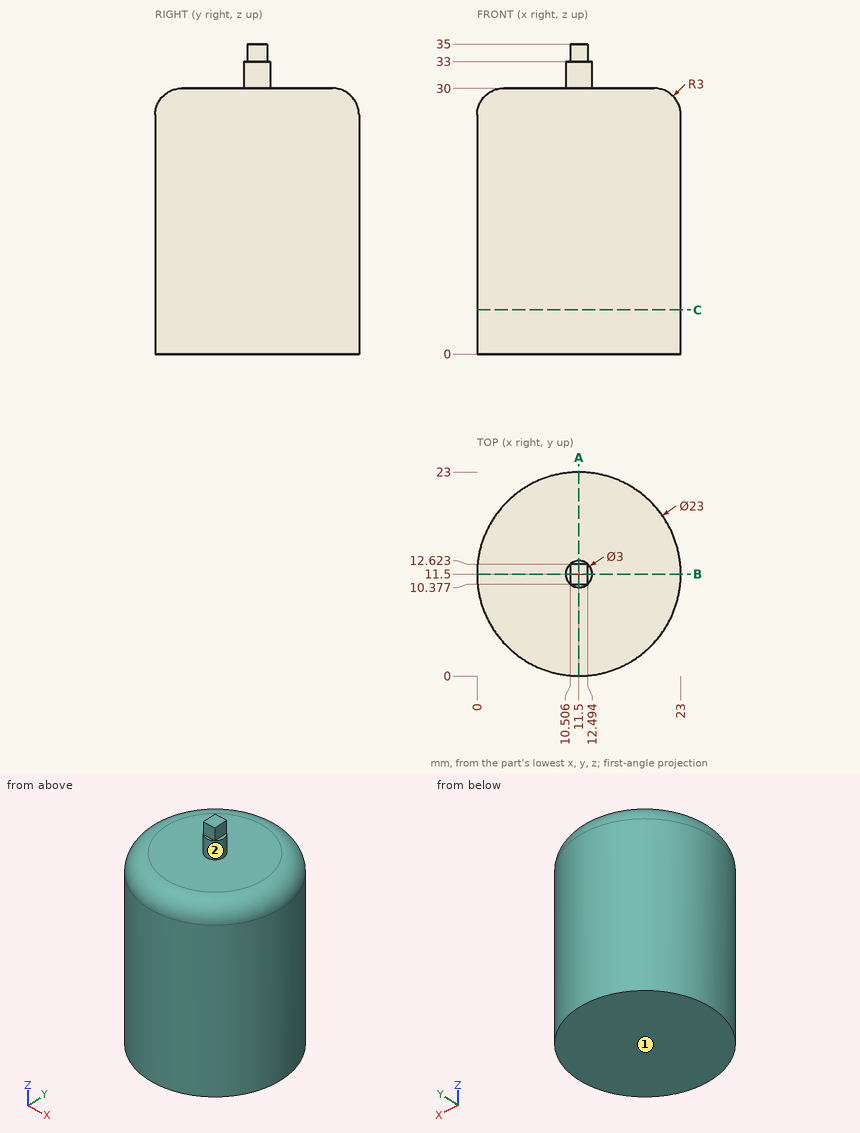
Here's the drawing with two shaded views (mm, measured from the low corner). I have some questions. A direction names the side the tool comes from. Give positions to 0.01 mm unless a question says otherwise; leave off trailing zeros. Order: outer loops, then holes, each group sorted by start corner. A loop starts at its lowest first (then second) coordinate and runs counter-clockwise, first axis right, second up. Notation, with made-up numbers: M -15.5,14.5 L 34.5,14.5 A9 ccw 34.5,23.5 Z; hole C 3.5,63 d7. An arc over 180 degrees is marked long. Answer as a JSON object with one key per item and string values. Group by question number.
1) Suppose I cut it at C-C, the plane z = 5. Write out the boundary of the cut face in (x, y).
2) Please list where these lines run through material, in increasing order: L1, parallel to Z at x = 11.5, y = 4.5; L2, parallel to X at y = 16.75, z = 4; L3, parallel to Y at x = 8, z = 19 (1 decimal). Write a range as [from, to].
3) On a 3-axis mill with a long thin cutter (end or side, diameter ignored), from which of +Z, -Z, +X, -X, +Y, -Y can I reach the whole of each face in a straight line? I mean the marked faces 1 and 2. Say none if no direction works.
4) Suppose I cut it at B-B, the plane y = 11.5. Write out the boundary of the cut face in (x, z).
5) Suppose I cut it at A-A, the plane x = 11.5. Write out the boundary of the cut face in (y, z).
6) I'm going to push flat-ended pins straight in: pin 1 Ø2 at (x, z) = (17.5, 6) entering from +Y (1 decimal); pin 2 Ø2 at (x, y) = (19, 18) entering from -Z; pin 3 Ø0.6 at (y, z) = (12, 33.5) entering from -X; pin 4 Ø1 at (y, z) = (6.5, 21) entering from +X. Where does each tip first touch, or does it pass through?
Results found:
{
 "1": {"outline": "C 11.5,11.5 d23"},
 "2": {"L1": "[0, 30]", "L2": "[1.27, 21.73]", "L3": "[0.5, 22.5]"},
 "3": {"face 1": "-Z, +X, -X, +Y, -Y", "face 2": "+Z"},
 "4": {"outline": "M 0,0 L 23,0 L 23,27 A3 ccw 20,30 L 13,30 L 13,33 L 12.49,33 L 12.49,35 L 10.51,35 L 10.51,33 L 10,33 L 10,30 L 3,30 A3 ccw 0,27 Z"},
 "5": {"outline": "M 0,0 L 23,0 L 23,27 A3 ccw 20,30 L 13,30 L 13,33 L 12.62,33 L 12.62,35 L 10.38,35 L 10.38,33 L 10,33 L 10,30 L 3,30 A3 ccw 0,27 Z"},
 "6": {"pin 1": "y = 21.9", "pin 2": "z = 0", "pin 3": "x = 10.51", "pin 4": "x = 22.08"}
}
